The drawing under review shows one solid part. Ordinate dimensions are in mm from its lowest x, y, z. A direction names the side the tool comes from. Give positions to 0.01 mm unless a question says otherwise; leave off trailing zeros. Loops run counter-clockwise (first coordinate to the right, second up) from the corner with the lowest first, then second, coordinate; pieces in that order, holes last. Notation, with made-up numbers: (-25, -32.5) -> (-9, -32.5) arc R6 cw to (-9, -22.5) -> close; hole circle Ø4 at (67.25, 13.25). An arc over 180 degrees is marked (long way). Answer in a Markdown table with one row per item. Add a question column.
(1) Consider section D-D on z = 61.5. Write out the cut boundary in (x, y).
(2) Consider section B-B on x = 8.65. Write out the cut boundary in (y, z), then the cut area to 4 significant figures.
(3) Consider section A-A on z = 20. Write out the cut boundary in (x, y).
(4) Consider section C-C on y = 18.5. Write out the cut boundary in (x, z).
(5) For pin 1 (4.5 mm diameter, centred on y = 18.5, z = 58.5, fed in from -X); pin 2 (1 mm diameter, centred on x = 104.5, z = 9, fed in from -Y); pin 3 (11.5 mm diameter, centred on x = 158.65, z = 20, fed in from +Y), all flat-tipped, find the tip position at first contact; note any pin that passes through.
(6) Draft analysis for pull direction X (two halves, no side actions). For the marked faces 4, 5 and 6, state which applies: +X half, -X half, draft (parallel to the pull), parting line (faces both ways), or undercut.
(7) For the marked faces 1, 2 and 3, list the 3-axis set-ups (+Z, -Z, +X, -X, +Y, -Y) from which the entire face can be reached by the end or side of a thin tool; tool diameter is ignored.
(8) For line 1 (Z direction, x = 120.95, y = 31); line 2 (X direction, y = 3.75, z = 20); line 3 (X direction, y = 1, z = 70), list the stretches that pass through material, from the lowest coordinate up.
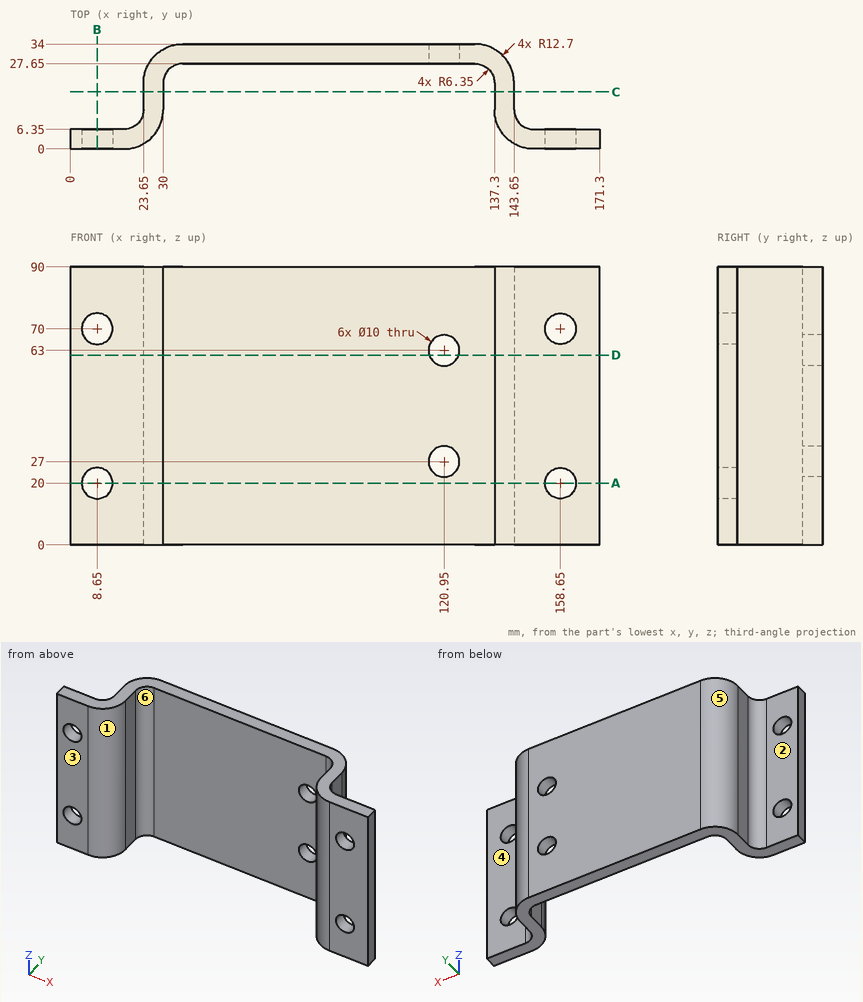
Values follow:
| question | item | result |
|---|---|---|
| 1 | outline | (0, 0) -> (17.3, 0) arc R12.7 ccw to (30, 12.7) -> (30, 21.3) arc R6.35 cw to (36.35, 27.65) -> (116.18, 27.65) -> (116.18, 34) -> (36.35, 34) arc R12.7 ccw to (23.65, 21.3) -> (23.65, 12.7) arc R6.35 cw to (17.3, 6.35) -> (0, 6.35) -> close; (125.72, 27.65) -> (130.95, 27.65) arc R6.35 cw to (137.3, 21.3) -> (137.3, 12.7) arc R12.7 ccw to (150, 0) -> (171.3, 0) -> (171.3, 6.35) -> (150, 6.35) arc R6.35 cw to (143.65, 12.7) -> (143.65, 21.3) arc R12.7 ccw to (130.95, 34) -> (125.72, 34) -> close |
| 2 | outline | (0, 0) -> (6.35, 0) -> (6.35, 15) -> (0, 15) -> close; (0, 25) -> (6.35, 25) -> (6.35, 65) -> (0, 65) -> close; (0, 75) -> (6.35, 75) -> (6.35, 90) -> (0, 90) -> close |
| 2 | area | 444.5 mm2 |
| 3 | outline | (0, 0) -> (3.65, 0) -> (3.65, 6.35) -> (0, 6.35) -> close; (13.65, 0) -> (17.3, 0) arc R12.7 ccw to (30, 12.7) -> (30, 21.3) arc R6.35 cw to (36.35, 27.65) -> (130.95, 27.65) arc R6.35 cw to (137.3, 21.3) -> (137.3, 12.7) arc R12.7 ccw to (150, 0) -> (153.65, 0) -> (153.65, 6.35) -> (150, 6.35) arc R6.35 cw to (143.65, 12.7) -> (143.65, 21.3) arc R12.7 ccw to (130.95, 34) -> (36.35, 34) arc R12.7 ccw to (23.65, 21.3) -> (23.65, 12.7) arc R6.35 cw to (17.3, 6.35) -> (13.65, 6.35) -> close; (163.65, 0) -> (171.3, 0) -> (171.3, 6.35) -> (163.65, 6.35) -> close |
| 4 | outline | (23.65, 0) -> (30, 0) -> (30, 90) -> (23.65, 90) -> close; (137.3, 0) -> (143.65, 0) -> (143.65, 90) -> (137.3, 90) -> close |
| 5 | pin 1 | x = 23.65 |
| 5 | pin 2 | y = 27.65 |
| 5 | pin 3 | y = 6.35 |
| 6 | face 4 | draft |
| 6 | face 5 | -X half |
| 6 | face 6 | undercut |
| 7 | face 1 | +Z, -Z, -Y |
| 7 | face 2 | +Z, -Z, -X, +Y |
| 7 | face 3 | +Z, -Z, +X, -X, -Y |
| 8 | line 1 | 0 to 22, 32 to 58, 68 to 90 |
| 8 | line 2 | 0 to 3.65, 13.65 to 26.31, 140.99 to 153.65, 163.65 to 171.3 |
| 8 | line 3 | 0 to 3.65, 13.65 to 22.24, 145.06 to 153.65, 163.65 to 171.3 |
